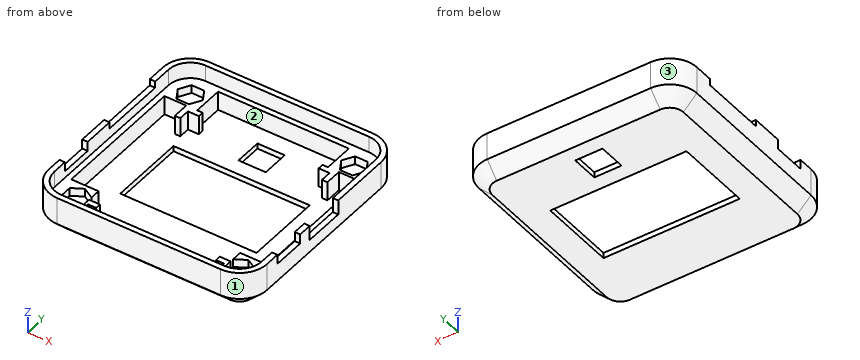
```python
from build123d import *

# Parameters (mm, degrees)
EXTRUDE_1_DEPTH     = 1
SKETCH_3_W          = 25
SKETCH_3_H          = 14
CUT_EXTRUDE_1_DEPTH = 30.381116385
EXTRUDE_START       = 6.5
EXTRUDE_2_DEPTH     = 6.5
EXTRUDE_START_2     = 3.5
EXTRUDE_3_DEPTH     = 3.5
EXTRUDE_4_DEPTH     = 3.5
CHAMFER_1_SIZE      = 2.5
EXTRUDE_5_DEPTH     = 3.5
EXTRUDE_6_DEPTH     = 3.5
CUT_EXTRUDE_2_DEPTH = 1.5
CUT_EXTRUDE_3_DEPTH = 1.5
CUT_EXTRUDE_4_REACH = 47.588
SKETCH_12_W         = 1.75
SKETCH_12_H         = 6
SKETCH_12_W_2       = 2.7
SKETCH_12_H_2       = 7.5
CUT_EXTRUDE_5_REACH = 47.588
SKETCH_13_W         = 1.2
SKETCH_13_H         = 12
SKETCH_14_W         = 5
SKETCH_14_H         = 5
CUT_EXTRUDE_6_DEPTH = 1.5
SKETCH_12_2_W       = 1.75
SKETCH_12_2_H       = 6
CUT_EXTRUDE_7_DEPTH = 46.587827323


with BuildPart() as part:
    # 草圖2 → 填料-伸長1 (new body)
    with BuildSketch(Plane(origin=(0, 0, -2.5), x_dir=(-1, 0, 0), z_dir=(0, 0, -1))):
        with BuildLine():
            Line((-15, -18.5), (15, -18.5))
            ThreePointArc((15, -18.5), (18.535533906, -17.035533906), (20, -13.5))
            Line((20, -13.5), (20, 16.5))
            ThreePointArc((20, 16.5), (18.535533906, 20.035533906), (15, 21.5))
            Line((15, 21.5), (-15, 21.5))
            ThreePointArc((-15, 21.5), (-18.535533906, 20.035533906), (-20, 16.5))
            Line((-20, 16.5), (-20, -13.5))
            ThreePointArc((-20, -13.5), (-18.535533906, -17.035533906), (-15, -18.5))
        make_face()
    extrude(amount=EXTRUDE_1_DEPTH)

    # 草圖3 → 除料-伸長1 (cut, through all)
    with BuildSketch(Plane(origin=(0, 0, -3.5), x_dir=(-1, 0, 0), z_dir=(0, 0, -1))):
        with Locations((0, 1.5)):
            Rectangle(SKETCH_3_W, SKETCH_3_H)
    extrude(amount=-CUT_EXTRUDE_1_DEPTH, mode=Mode.SUBTRACT)

    # 草圖4 → 填料-伸長2 (add)
    with BuildSketch(Plane.XY.offset(-2.5).offset(EXTRUDE_START)):
        with BuildLine():
            Line((15, -18.5), (-15, -18.5))
            ThreePointArc((-15, -18.5), (-18.535533906, -17.035533906), (-20, -13.5))
            Line((-20, -13.5), (-20, 16.5))
            ThreePointArc((-20, 16.5), (-18.535533906, 20.035533906), (-15, 21.5))
            Line((-15, 21.5), (15, 21.5))
            ThreePointArc((15, 21.5), (18.535533906, 20.035533906), (20, 16.5))
            Line((20, 16.5), (20, -13.5))
            ThreePointArc((20, -13.5), (18.535533906, -17.035533906), (15, -18.5))
        make_face()
        with BuildLine():
            Line((19, -13.5), (19, 16.5))
            ThreePointArc((19, 16.5), (17.828427125, 19.328427125), (15, 20.5))
            Line((15, 20.5), (-15, 20.5))
            ThreePointArc((-15, 20.5), (-17.828427125, 19.328427125), (-19, 16.5))
            Line((-19, 16.5), (-19, -13.5))
            ThreePointArc((-19, -13.5), (-17.828427125, -16.328427125), (-15, -17.5))
            Line((-15, -17.5), (15, -17.5))
            ThreePointArc((15, -17.5), (17.828427125, -16.328427125), (19, -13.5))
        make_face(mode=Mode.SUBTRACT)
    extrude(amount=-EXTRUDE_2_DEPTH)

    # 草圖5 → 填料-伸長3 (add)
    with BuildSketch(Plane.XY.offset(-2.5).offset(EXTRUDE_START_2)):
        with BuildLine():
            Line((19, -13.5), (19, 16.5))
            ThreePointArc((19, 16.5), (17.828427125, 19.328427125), (15, 20.5))
            Line((15, 20.5), (-15, 20.5))
            ThreePointArc((-15, 20.5), (-17.828427125, 19.328427125), (-19, 16.5))
            Line((-19, 16.5), (-19, -13.5))
            ThreePointArc((-19, -13.5), (-17.828427125, -16.328427125), (-15, -17.5))
            Line((-15, -17.5), (15, -17.5))
            ThreePointArc((15, -17.5), (17.828427125, -16.328427125), (19, -13.5))
        make_face()
        with BuildLine():
            Line((18, -13.5), (18, 16.5))
            ThreePointArc((18, 16.5), (17.121320344, 18.621320344), (15, 19.5))
            Line((15, 19.5), (-15, 19.5))
            ThreePointArc((-15, 19.5), (-17.121320344, 18.621320344), (-18, 16.5))
            Line((-18, 16.5), (-18, -13.5))
            ThreePointArc((-18, -13.5), (-17.121320344, -15.621320344), (-15, -16.5))
            Line((-15, -16.5), (15, -16.5))
            ThreePointArc((15, -16.5), (17.121320344, -15.621320344), (18, -13.5))
        make_face(mode=Mode.SUBTRACT)
    extrude(amount=-EXTRUDE_3_DEPTH)

    # 草圖6 → 填料-伸長4 (add)
    with BuildSketch(Plane.XY.offset(-2.5)):
        Polygon((14, -14), (14, -10.5), (13, -10.5), (13, -13), (11, -13), (11, -14), align=None)
        Polygon((14, 14), (11, 14), (11, 13), (13, 13), (13, 11), (14, 11), align=None)
        Polygon((-14, 14), (-14, 11), (-13, 11), (-13, 13), (-11, 13), (-11, 14), align=None)
        Polygon((-14, -14), (-11, -14), (-11, -13), (-13, -13), (-13, -10.5), (-14, -10.5), align=None)
    extrude(amount=EXTRUDE_4_DEPTH)

    # 導角1
    chamfer_1_edges = [part.edges().sort_by_distance(p)[0] for p in [
        (18.535533906, -17.035533906, -3.5),
        (0, -18.5, -3.5),
        (-18.535533906, -17.035533906, -3.5),
        (-20, 1.5, -3.5),
        (-18.535533906, 20.035533906, -3.5),
        (0, 21.5, -3.5),
        (18.535533906, 20.035533906, -3.5),
        (20, 1.5, -3.5),
    ]]
    chamfer(chamfer_1_edges, length=CHAMFER_1_SIZE)

    # 草圖7 → 填料-伸長5 (add)
    with BuildSketch(Plane.XY.offset(-2.5).offset(EXTRUDE_START_2)):
        with BuildLine():
            Line((-12, 19.5), (-12, 14))
            Line((-12, 14), (-18, 14))
            Line((-18, 14), (-18, 16.5))
            ThreePointArc((-18, 16.5), (-17.121320344, 18.621320344), (-15, 19.5))
            Line((-15, 19.5), (-12, 19.5))
        make_face()
    extrude_5 = extrude(amount=-EXTRUDE_5_DEPTH)

    # 草圖8 → 填料-伸長6 (add)
    with BuildSketch(Plane.XY.offset(-2.5).offset(EXTRUDE_START_2)):
        with BuildLine():
            Line((-12.5, -16.5), (-12.5, -14))
            Line((-12.5, -14), (-14, -14))
            Line((-14, -14), (-14, -10.5))
            Line((-14, -10.5), (-18, -10.5))
            Line((-18, -10.5), (-18, -13.5))
            ThreePointArc((-18, -13.5), (-17.121320344, -15.621320344), (-15, -16.5))
            Line((-15, -16.5), (-12.5, -16.5))
        make_face()
    extrude_6 = extrude(amount=-EXTRUDE_6_DEPTH)

    # 鏡射2: 填料-伸長5, 填料-伸長6 across plane
    add(extrude_5.mirror(Plane(origin=(0, 0, 0), x_dir=(0, 0, 1), z_dir=(1, 0, 0))))
    add(extrude_6.mirror(Plane(origin=(0, 0, 0), x_dir=(0, 0, 1), z_dir=(1, 0, 0))))

    # 草圖10 → 除料-伸長2 (cut)
    with BuildSketch(Plane.XY.offset(1)):
        Polygon((-15, -15.809401077), (-13, -14.654700538), (-13, -12.345299462), (-15, -11.190598923), (-17, -12.345299462), (-17, -14.654700538), align=None)
    cut_extrude_2 = extrude(amount=-CUT_EXTRUDE_2_DEPTH, mode=Mode.SUBTRACT)

    # 草圖11 → 除料-伸長3 (cut)
    with BuildSketch(Plane.XY.offset(1)):
        Polygon((-17.309401077, 16.5), (-16.154700538, 14.5), (-13.845299462, 14.5), (-12.690598923, 16.5), (-13.845299462, 18.5), (-16.154700538, 18.5), align=None)
    cut_extrude_3 = extrude(amount=-CUT_EXTRUDE_3_DEPTH, mode=Mode.SUBTRACT)

    # 鏡射3: 除料-伸長2, 除料-伸長3 across plane
    add(cut_extrude_2.mirror(Plane(origin=(0, 0, 0), x_dir=(0, 0, 1), z_dir=(1, 0, 0))), mode=Mode.SUBTRACT)
    add(cut_extrude_3.mirror(Plane(origin=(0, 0, 0), x_dir=(0, 0, 1), z_dir=(1, 0, 0))), mode=Mode.SUBTRACT)

    # 草圖12 → 除料-伸長4 (cut, up to next)
    with BuildSketch(Plane(origin=(20, 0, 0), x_dir=(0, 0, -1), z_dir=(1, 0, 0)), mode=Mode.PRIVATE) as cut_extrude_4_sk1:
        with Locations((-3.125, -7.75)):
            Rectangle(SKETCH_12_W, SKETCH_12_H)
    cut_extrude_4_tool1 = extrude(cut_extrude_4_sk1.sketch, amount=-CUT_EXTRUDE_4_REACH, mode=Mode.PRIVATE) & part.part
    # 草圖12 → 除料-伸長4 (cut, up to next)
    with BuildSketch(Plane(origin=(20, 0, 0), x_dir=(0, 0, -1), z_dir=(1, 0, 0)), mode=Mode.PRIVATE) as cut_extrude_4_sk2:
        with Locations((-2.65, 1.5)):
            Rectangle(SKETCH_12_W_2, SKETCH_12_H_2)
    cut_extrude_4_tool2 = extrude(cut_extrude_4_sk2.sketch, amount=-CUT_EXTRUDE_4_REACH, mode=Mode.PRIVATE) & part.part
    add(cut_extrude_4_tool1.solids().sort_by_distance((20, -7.75, 3.125))[0], mode=Mode.SUBTRACT)
    add(cut_extrude_4_tool2.solids().sort_by_distance((20, 1.5, 2.65))[0], mode=Mode.SUBTRACT)

    # 草圖13 → 除料-伸長5 (cut, up to next)
    with BuildSketch(Plane.ZY.offset(20), mode=Mode.PRIVATE) as cut_extrude_5_sk1:
        with Locations((3.4, 7)):
            Rectangle(SKETCH_13_W, SKETCH_13_H)
    cut_extrude_5_tool1 = extrude(cut_extrude_5_sk1.sketch, amount=-CUT_EXTRUDE_5_REACH, mode=Mode.PRIVATE) & part.part
    add(cut_extrude_5_tool1.solids().sort_by_distance((-20, 7, 3.4))[0], mode=Mode.SUBTRACT)

    # 草圖14 → 除料-伸長6 (cut)
    with BuildSketch(Plane(origin=(0, 0, -3.5), x_dir=(-1, 0, 0), z_dir=(0, 0, -1))):
        with Locations((0, 13.75)):
            Rectangle(SKETCH_14_W, SKETCH_14_H)
    extrude(amount=-CUT_EXTRUDE_6_DEPTH, mode=Mode.SUBTRACT)

    # 草圖12<2> → 除料-伸長7 (cut, through all)
    with BuildSketch(Plane(origin=(20, 0, 0), x_dir=(0, 0, -1), z_dir=(1, 0, 0))):
        with Locations((-3.125, -7.75)):
            Rectangle(SKETCH_12_2_W, SKETCH_12_2_H)
    extrude(amount=-CUT_EXTRUDE_7_DEPTH, mode=Mode.SUBTRACT)


solid = part.part
```
Can you work these out from the model? Positions are in its coordinate system, mm. Face numbers are marked on the shaded views. Coordinates: 2 decimals unless noted, no trailing zeros. Loops run counter-clockwise (first coordinate to the right, second up) from the corner with the lowest first, then second, coordinate; pieces in that order, holes last. Notation, with made-up numbers: M -20.75,81.5 L 20.25,81.5 A17 cw 20.25,110.5 Z; hole C 9,7.25 d1. An arc over 180 degrees is marked long. Put each result on its own line as item: value. Start each with the question number.
(1) Imagine slicing it at B-B on y = -4. List the corners of the cut face in (x, z) for me, and give its area (4 significant figures).
(2) Will these pins go through, and if not, where does the flat tip stop? pin 1 Ø10 at (x, y) = (-0.5, 15) entering from +Z; pin 2 Ø2 at (y, z) = (-15.5, -1) entering from +X; pin 3 Ø1 at (x, y) = (-2.5, 14) entering from +Z.
(3) I need wall thicknesses on probe 1 along Y at (x, z) = (-9, 2.5); probe 2 along Y at (x, z) = (9, -1); probe 3 along X at (y, z) = (-1, -3). Which ranges of each line are inside material? Lowest first, please.
(4) Imagine slicing it at D-D on y = 12.5. List the corners of the cut face in (x, z) for me, and give its area (4 significant figures).
(5) Imagine slicing it at C-C on x = -11.5. List the corners of the cut face in (y, z) for me, and give its area (4 significant figures).
(6) Imagine slicing it at A-A on x = -0.5. List the corners of the cut face in (y, z) for me.
(7) We'd pull the mould along Y, two halves only. Please class the marked faces 1, 2 and 3: +Y half, -Y half, draft (parallel to the pull), parting line (faces both ways), or undercut.
Worked answers:
1. outline: M -20,-1 L -17.5,-3.5 L -12.5,-3.5 L -12.5,-2.5 L -18,-2.5 L -18,1 L -19,1 L -19,4 L -20,4 Z; M 12.5,-3.5 L 17.5,-3.5 L 20,-1 L 20,4 L 19,4 L 19,1 L 18,1 L 18,-2.5 L 12.5,-2.5 Z
1. area: 28.75 mm2
2. pin 1: stops at z = 1
2. pin 2: stops at x = 19.9
2. pin 3: stops at z = -2.5
3. probe 1: y = -18.5 to -17.5, 20.5 to 21.5
3. probe 2: y = -18.5 to -16.5, 19.5 to 21.5
3. probe 3: x = -18 to -12.5, 12.5 to 18
4. outline: M -20,-1 L -17.5,-3.5 L -2.5,-3.5 L -2.5,-2.5 L -13,-2.5 L -13,1 L -14,1 L -14,-2.5 L -18,-2.5 L -18,1 L -19,1 L -19,2.8 L -20,2.8 Z; M 2.5,-3.5 L 17.5,-3.5 L 20,-1 L 20,4 L 19,4 L 19,1 L 18,1 L 18,-2.5 L 14,-2.5 L 14,1 L 13,1 L 13,-2.5 L 2.5,-2.5 Z
4. area: 54.55 mm2
5. outline: M -18.5,-1 L -16,-3.5 L -5.5,-3.5 L -5.5,-2.5 L -13,-2.5 L -13,1 L -14,1 L -14,-2.5 L -16.5,-2.5 L -16.5,1 L -17.5,1 L -17.5,4 L -18.5,4 Z; M 8.5,-3.5 L 19,-3.5 L 21.5,-1 L 21.5,4 L 20.5,4 L 20.5,1 L 19.5,1 L 19.5,-2.5 L 14,-2.5 L 14,1 L 13,1 L 13,-2.5 L 8.5,-2.5 Z
5. area: 46.75 mm2
6. outline: M -18.5,-1 L -16,-3.5 L -5.5,-3.5 L -5.5,-2.5 L -16.5,-2.5 L -16.5,1 L -17.5,1 L -17.5,4 L -18.5,4 Z; M 8.5,-3.5 L 11.25,-3.5 L 11.25,-2.5 L 8.5,-2.5 Z; M 16.25,-3.5 L 19,-3.5 L 21.5,-1 L 21.5,4 L 20.5,4 L 20.5,1 L 19.5,1 L 19.5,-2.5 L 16.25,-2.5 Z
7. face 1: -Y half
7. face 2: undercut
7. face 3: +Y half
